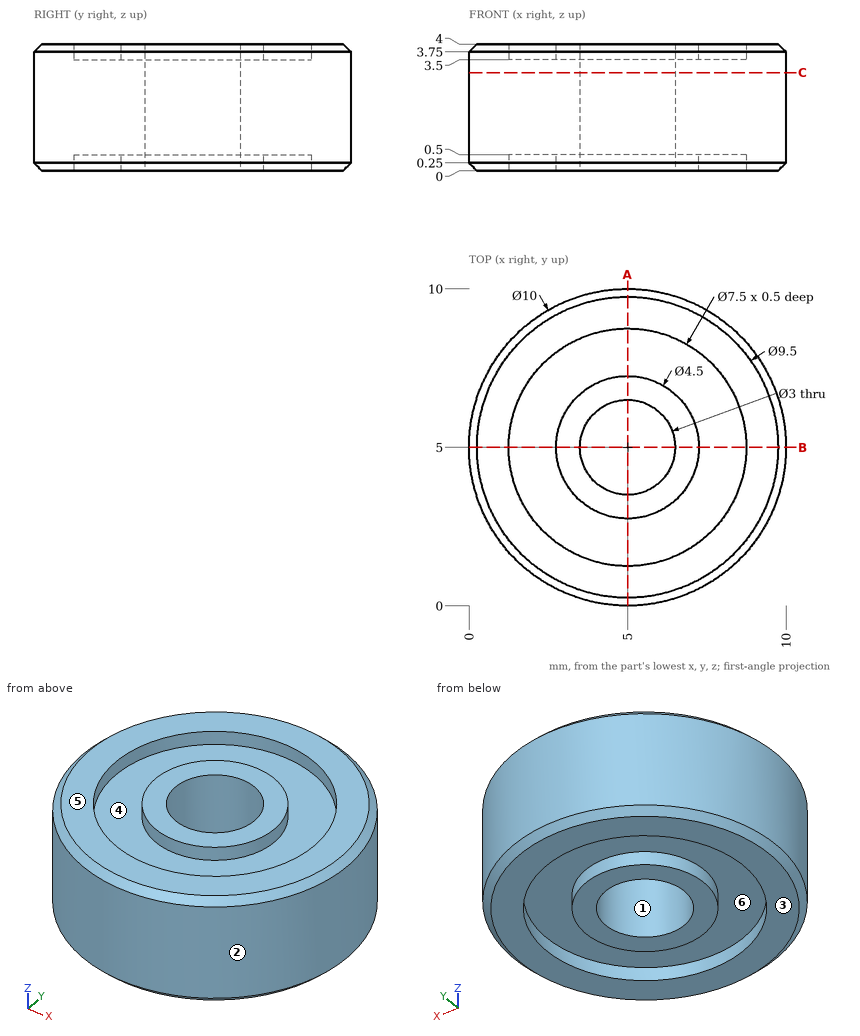
Study the drawing (mm; zero at the part's minimum x, y, z) and answer. A direction names the side the tool comes from. Coordinates: 2 decimals unless noted, no trailing zeros. Order: outer loops, then holes, each group sorted by start corner. A loop starts at its lowest first (then second) coordinate and runs counter-clockwise, first axis right, second up. Notation, with made-up numbers: M 63.25,63.5 L 118.25,63.5 A11 cw 118.25,72.5 Z; hole C 65,15.25 d3. An arc over 180 degrees is marked long. Answer as a JSON object with one key per item and string values. Group by question number.
1. Straight lines are drawn through the part: line 1 (X direction, y = 5, z = 3.7); line 2 (Y direction, x = 5, z = 2.25). For each, find the intervals that lie inside material, in ascending order.
2. Section C-C on z = 3.1 is taken. Write down the section's boundary in (x, y).
3. A tool of negligible diameter and unlimited length cuts with its end or side. For the marked faces 4, 5 and 6, from which of +Z, -Z, +X, -X, +Y, -Y can it reach the whole face along a straight path? Write none if from no direction.
4. Flat-ended cylindrical pins translate along their axes: P1, Ø1.5, axis at x = 3, z = 3, coming from the +Y side; P2, Ø2.5, axis at x = 5, y = 5, coming from the +Z side. Find the tip coordinate at first contact, or state that the pin passes through.
5. Section A-A on x = 5 is taken. Write down the section's boundary in (y, z).
6. Determine the mould class of the marked faces 1, 2 and 3 for opening direction Y: released by +Y, released by -Y, zero draft, split by the parting line, or undercut.
Values follow:
{
 "1": {"line 1": "0 to 1.25, 2.75 to 3.5, 6.5 to 7.25, 8.75 to 10", "line 2": "0 to 3.5, 6.5 to 10"},
 "2": {"outline": "C 5,5 d10; hole C 5,5 d3"},
 "3": {"face 4": "+Z", "face 5": "+Z, +X, -X, +Y, -Y", "face 6": "-Z"},
 "4": {"P1": "y = 9.84", "P2": "through"},
 "5": {"outline": "M 0,0.25 L 0.25,0 L 1.25,0 L 1.25,0.5 L 2.75,0.5 L 2.75,0 L 3.5,0 L 3.5,4 L 2.75,4 L 2.75,3.5 L 1.25,3.5 L 1.25,4 L 0.25,4 L 0,3.75 Z; M 6.5,0 L 7.25,0 L 7.25,0.5 L 8.75,0.5 L 8.75,0 L 9.75,0 L 10,0.25 L 10,3.75 L 9.75,4 L 8.75,4 L 8.75,3.5 L 7.25,3.5 L 7.25,4 L 6.5,4 Z"},
 "6": {"face 1": "undercut", "face 2": "split by the parting line", "face 3": "zero draft"}
}
